Drawing for the job (mm, zero at the part's lowest x, y, z). Give positions to 0.01 mm unless a question says otherwise; leave off trailing zeros. Write each loop counter-clockwise with the first axis right and the second up, starting at its lowest first coordinate (ties: lowest second). Pieces come first, ordered by that corner, then holes. Notation, with made-up numbers: (-31.75, 45.25) - (-17.75, 45.25) arc R12 ccw to (-17.75, 67.25) - close; hole circle Ø9 at (53.5, 34). An arc over 180 degrees is marked (long way). Use CSV: the item, a comma, the result in double quotes.
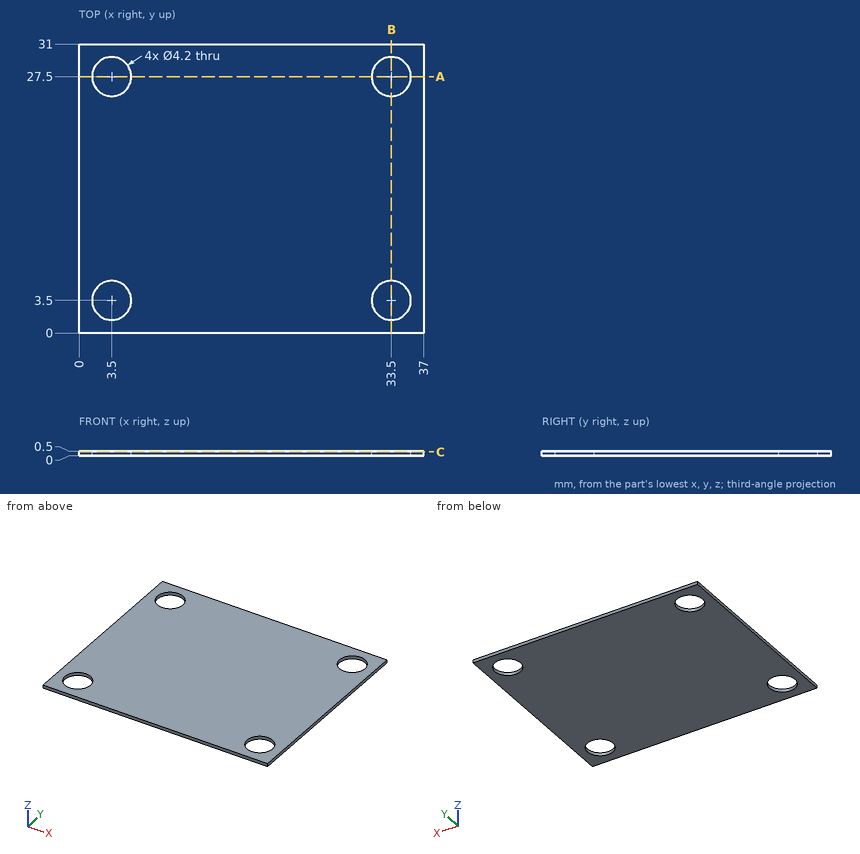
(1) Flat gauge pin, fed straight in: P1, Ø4, axis at x = 33.5, y = 3.5, coming from the -Z side. Where does the tip first touch, or does it go through?
Checked values:
P1,"passes through"
(2) Saw through at C-C, the plane z = 0.4. List the corners of the cut face in (x, y), then the cut area to 3 significant figures.
Checked values:
outline,"(0, 0) - (37, 0) - (37, 31) - (0, 31) - close; hole circle Ø4.2 at (3.5, 3.5); hole circle Ø4.2 at (3.5, 27.5); hole circle Ø4.2 at (33.5, 3.5); hole circle Ø4.2 at (33.5, 27.5)"
area,"1,090 mm^2"
(3) Saw through at A-A, the plane y = 27.5. List the corners of the cut face in (x, z), then the cut area to 3 significant figures.
Checked values:
outline,"(0, 0) - (1.4, 0) - (1.4, 0.5) - (0, 0.5) - close; (5.6, 0) - (31.4, 0) - (31.4, 0.5) - (5.6, 0.5) - close; (35.6, 0) - (37, 0) - (37, 0.5) - (35.6, 0.5) - close"
area,"14.3 mm^2"
(4) Wall check: probe 1 along X at (y, z) = (27.5, 0.15); probe 2 along Y at (x, z) = (33.5, 0.35); probe 3 along X at (y, z) = (26.5, 0.4). Give the ranges that are in metal, low to high. Write a range as [from, to].
Checked values:
probe 1,"x = [0, 1.4], [5.6, 31.4], [35.6, 37]"
probe 2,"y = [0, 1.4], [5.6, 25.4], [29.6, 31]"
probe 3,"x = [0, 1.65], [5.35, 31.65], [35.35, 37]"
(5) Saw through at B-B, the plane x = 33.5. List the corners of the cut face in (y, z).
Checked values:
outline,"(0, 0) - (1.4, 0) - (1.4, 0.5) - (0, 0.5) - close; (5.6, 0) - (25.4, 0) - (25.4, 0.5) - (5.6, 0.5) - close; (29.6, 0) - (31, 0) - (31, 0.5) - (29.6, 0.5) - close"
